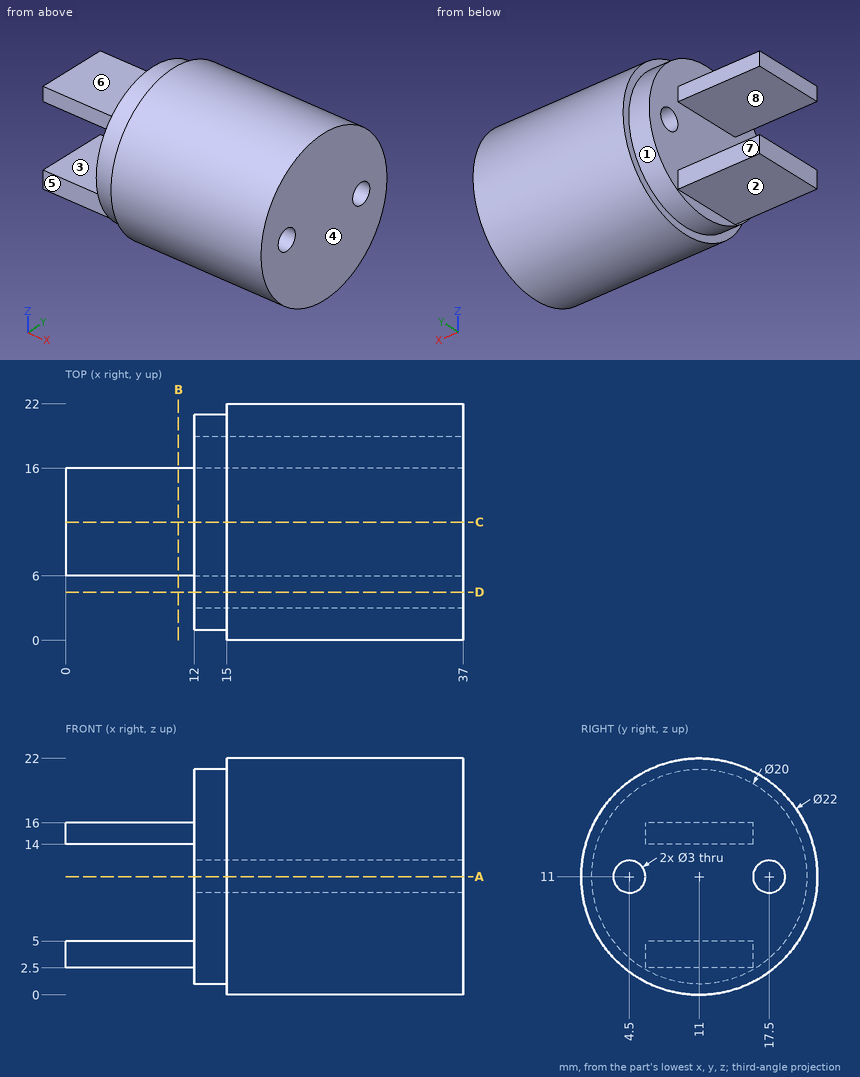
Design review of the part shown in the three views and the two pictorial views. Dimensions are in mm from the part's minimum x, y and z. A direction names the side the tool comes from. Give positions to 0.01 mm unless a question says otherwise; leave off trailing zeros. Loops run counter-clockwise (first coordinate to the right, second up) from the corner with the lowest first, then second, coordinate; pieces in that order, holes last. Notation, with made-up numbers: (6, -6) -> (32, -6) arc R17 ccw to (32, 13) -> close; hole circle Ø11 at (44.25, 23). An arc over 180 degrees is marked (long way). Answer as a JSON object with one key per item and string values. Group by question number.
Q1. Take a section at C-C (y = 11). Write out the cut boundary in (x, z), plus the area to 3 significant figures.
Q2. Take a section at B-B (x = 10.5). Write out the cut boundary in (y, z), plus the area to 3 significant figures.
Q3. Insertion check: pin 1 (8 mm diameter, centred on x = 14, z = 20, fed in from +Y); pin 2 (1 mm diameter, centred on x = 22, z = 14, fed in from -Y); pin 3 (0.8 mm diameter, centred on x = 3.5, z = 3.5, fed in from +Y). Each pin has a flat end and moves straight along its axis. Give the tip position at first contact, or say it passes through.
Q4. Wall thickness on line 1 along Z through (x, y) = (2, 12); line 2 along X through (y, z) = (19.75, 9); line 3 along Z through (x, y) = (27.5, 17.5): over which ranges is each line inside the solid? List them lowest first.
Q5. Take a section at A-A (z = 11). Write out the cut boundary in (x, y).
Q6. Take a section at D-D (y = 4.5). Write out the cut boundary in (x, z), plus the area to 3 significant figures.
Q7. Tool access review of the marked faces 5, 6, 7 and 8: name each direction out of +Z, -Z, +X, -X, +Y, -Y from which nothing blocks a thin tool from reaching the whole face with its end or side.
Q8. Draft analysis for pull direction Z (two halves, no side actions). For the marked faces 1, 2, 3 and 4, state which applies: pulls with the +Z half, pulls with the -Z half, needs draft (parallel to the pull), parting line crosses it, or undercut.
Answer below:
{
 "1": {"outline": "(0, 2.5) -> (12, 2.5) -> (12, 1) -> (15, 1) -> (15, 0) -> (37, 0) -> (37, 22) -> (15, 22) -> (15, 21) -> (12, 21) -> (12, 16) -> (0, 16) -> (0, 14) -> (12, 14) -> (12, 5) -> (0, 5) -> close", "area": "598 mm2"},
 "2": {"outline": "(6, 2.5) -> (16, 2.5) -> (16, 5) -> (6, 5) -> close; (6, 14) -> (16, 14) -> (16, 16) -> (6, 16) -> close", "area": "45.0 mm2"},
 "3": {"pin 1": "stops at y = 20.73", "pin 2": "stops at y = 0.29", "pin 3": "stops at y = 16"},
 "4": {"line 1": "z = 2.5 to 5, 14 to 16", "line 2": "x = 12 to 37", "line 3": "z = 2.13 to 9.5, 12.5 to 19.87"},
 "5": {"outline": "(12, 1) -> (15, 1) -> (15, 0) -> (37, 0) -> (37, 3) -> (12, 3) -> close; (12, 6) -> (37, 6) -> (37, 16) -> (12, 16) -> close; (12, 19) -> (37, 19) -> (37, 22) -> (15, 22) -> (15, 21) -> (12, 21) -> close"},
 "6": {"outline": "(12, 3.4) -> (15, 3.4) -> (15, 2.13) -> (37, 2.13) -> (37, 9.5) -> (12, 9.5) -> close; (12, 12.5) -> (37, 12.5) -> (37, 19.87) -> (15, 19.87) -> (15, 18.6) -> (12, 18.6) -> close", "area": "361 mm2"},
 "7": {"face 5": "+Z, -Z, -X, -Y", "face 6": "+Z, -X, +Y, -Y", "face 7": "+Z, -Z, -X, +Y", "face 8": "-X, +Y, -Y"},
 "8": {"face 1": "parting line crosses it", "face 2": "pulls with the -Z half", "face 3": "undercut", "face 4": "needs draft"}
}
